from build123d import *

# Parameters (mm, degrees)
BOSS_EXTRUDE1_DEPTH                               = 3
CONVERT_SOLID1_DEPTH                              = 1
SKETCH8_R                                         = 2
CUT_EXTRUDE1_DEPTH                                = 2
CSK_FOR_4_FLAT_HEAD_MACHINE_SCREW_100_D           = 3.2639
CSK_FOR_4_FLAT_HEAD_MACHINE_SCREW_100_DEPTH       = 2
CSK_FOR_4_FLAT_HEAD_MACHINE_SCREW_100_CSINK_D     = 5.715
CSK_FOR_4_FLAT_HEAD_MACHINE_SCREW_100_CSINK_ANGLE = 100
CSK_FOR_4_FLAT_HEAD_MACHINE_SCREW_100_TIP         = 0.980574487


# Read off the part's stored shape, not the designer's step: Convert-Solid1
with BuildPart() as part:
    # Sketch2 → Boss-Extrude1 (new body)
    with BuildSketch(Plane(origin=(0, 0, 0), x_dir=(1, 0, 0), z_dir=(0, 1, 0))):
        with BuildLine():
            Line((-15.860247962, 17.20906431), (-13.637639272, 20.383278482))
            ThreePointArc((-13.637639272, 20.383278482), (-19.875283017, 22.35), (-26.112926762, 20.383278482))
            Line((-26.112926762, 20.383278482), (-26.112926762, 33.35))
            Line((-26.112926762, 33.35), (-26.112926762, 55.85))
            Line((-26.112926762, 55.85), (-16.112926762, 55.85))
            Line((-16.112926762, 55.85), (-16.112926762, 33.35))
            Line((-16.112926762, 33.35), (26.112926762, 33.35))
            Line((26.112926762, 33.35), (26.112926762, 20.383278482))
            ThreePointArc((26.112926762, 20.383278482), (19.875283017, 22.35), (13.637639272, 20.383278482))
            Line((13.637639272, 20.383278482), (15.860247962, 17.20906431))
            ThreePointArc((15.860247962, 17.20906431), (13.666207185, 14.707240293), (12.875283017, 11.475))
            ThreePointArc((12.875283017, 11.475), (10.092914311, 8.804356775), (6.237643745, 8.908278482))
            ThreePointArc((6.237643745, 8.908278482), (0, 10.875), (-6.237643745, 8.908278482))
            ThreePointArc((-6.237643745, 8.908278482), (-10.092914311, 8.804356775), (-12.875283017, 11.475))
            ThreePointArc((-12.875283017, 11.475), (-13.666207185, 14.707240293), (-15.860247962, 17.20906431))
        make_face()
    extrude(amount=BOSS_EXTRUDE1_DEPTH)

    # Convert-Solid1 outline → Convert-Solid1 (cut)
    with BuildSketch(Plane(origin=(0, 0, 0), x_dir=(1, 0, 0), z_dir=(0, 1, 0))):
        with BuildLine():
            Line((-26.112926762, 55.85), (-26.112926762, 20.383278482))
            ThreePointArc((-26.112926762, 20.383278482), (-19.875283017, 22.35), (-13.637639272, 20.383278482))
            Line((-13.637639272, 20.383278482), (-15.860247962, 17.20906431))
            ThreePointArc((-15.860247962, 17.20906431), (-13.666207185, 14.707240292), (-12.875283017, 11.475))
            ThreePointArc((-12.875283017, 11.475), (-10.092914311, 8.804356775), (-6.237643745, 8.908278482))
            ThreePointArc((-6.237643745, 8.908278482), (0, 10.875), (6.237643745, 8.908278482))
            ThreePointArc((6.237643745, 8.908278482), (10.092914311, 8.804356775), (12.875283017, 11.475))
            ThreePointArc((12.875283017, 11.475), (13.666207185, 14.707240292), (15.860247962, 17.20906431))
            Line((15.860247962, 17.20906431), (13.637639272, 20.383278482))
            ThreePointArc((13.637639272, 20.383278482), (19.875283017, 22.35), (26.112926762, 20.383278482))
            Line((26.112926762, 20.383278482), (26.112926762, 33.35))
            Line((26.112926762, 33.35), (-16.112926762, 33.35))
            Line((-16.112926762, 33.35), (-16.112926762, 55.85))
            Line((-16.112926762, 55.85), (-26.112926762, 55.85))
        make_face()
    extrude(amount=CONVERT_SOLID1_DEPTH, mode=Mode.SUBTRACT)

    # Sketch8 → Cut-Extrude1 (cut)
    with BuildSketch(Plane(origin=(0, 3, 0), x_dir=(1, 0, 0), z_dir=(0, 1, 0))):
        with Locations(Location((-21.112926762, 51.85, 0), (0, 0, 270))):
            Circle(SKETCH8_R)
        with Locations(Location((-21.112926762, 42.35, 0), (0, 0, 270))):
            Circle(SKETCH8_R)
    extrude(amount=-CUT_EXTRUDE1_DEPTH, mode=Mode.SUBTRACT)

    # CSK for #4 Flat Head Machine Screw (100)1
    with Locations(Plane(origin=(0, 3, 0), x_dir=(1, 0, 0), z_dir=(0, 1, 0))):
        with Locations((7.875283017, 28.35), (-7.875283017, 28.35)):
            CounterSinkHole(CSK_FOR_4_FLAT_HEAD_MACHINE_SCREW_100_D / 2, CSK_FOR_4_FLAT_HEAD_MACHINE_SCREW_100_CSINK_D / 2, depth=CSK_FOR_4_FLAT_HEAD_MACHINE_SCREW_100_DEPTH, counter_sink_angle=CSK_FOR_4_FLAT_HEAD_MACHINE_SCREW_100_CSINK_ANGLE)
            with Locations((0, 0, -(CSK_FOR_4_FLAT_HEAD_MACHINE_SCREW_100_DEPTH + CSK_FOR_4_FLAT_HEAD_MACHINE_SCREW_100_TIP / 2))):  # 118° drill point
                Cone(0, CSK_FOR_4_FLAT_HEAD_MACHINE_SCREW_100_D / 2, CSK_FOR_4_FLAT_HEAD_MACHINE_SCREW_100_TIP, mode=Mode.SUBTRACT)


solid = part.part
Part model, mm, in its own coordinate system. A direction names the side the tool comes from. Give positions to 0.01 mm unless a question says otherwise; leave off trailing zeros. Write each loop counter-clockwise with the first axis right and the second up, starting at its lowest first coordinate (ties: lowest second). Pieces come first, ordered by that corner, then holes.
1) Cut at D-D on z = -35.5. Write the cut outline in (x, y), then the cut area to 3 significant figures.
Resolved:
outline: (-26.11, 1) - (-16.11, 1) - (-16.11, 3) - (-26.11, 3) - close
area: 20.0 mm2
2) Probe L1, parallel to X at y = 1.65, z = -28.35; L2, parallel to X at y = 1.6, z = -42.35; L3, parallel to X at y = 1.45, z = -21.5. List the from-to ranges inside material, lowest first.
Resolved:
L1: x = -26.11 to -9.51, -6.24 to 6.24, 9.51 to 26.11
L2: x = -26.11 to -23.11, -19.11 to -16.11
L3: x = -26.11 to -24.09, -15.66 to 15.66, 24.09 to 26.11
3) Which spindle directions (+Z, -Z, +X, -X, +Y, -Y) get a long thin tool onto all of the face, cutting with end or side? Do faces 1 (the face through (5, 2, -33.35)), 2 (the face through (14.73, 1.99, -18.82)), 3 (the face through (10.145, 1.986, -8.825)), 4 (the face through (19.97, 1.99, -22.35)). Say none if no direction does.
Resolved:
face 1: -Z, +X, +Y, -Y
face 2: +X, +Y, -Y
face 3: +Z, +Y, -Y
face 4: +Y, -Y
4) Cut at C-C on x = 4. Write the cut outline in (y, z), then the cut area to 3 significant figures.
Resolved:
outline: (1, -33.35) - (3, -33.35) - (3, -10.11) - (1, -10.11) - close
area: 46.5 mm2
5) Cut at B-B on z = -28.35. Write the cut outline in (x, y), then the cut area to 3 significant figures.
Resolved:
outline: (-26.11, 1) - (-9.51, 1) - (-9.51, 1.97) - (-10.73, 3) - (-26.11, 3) - close; (-6.24, 1) - (6.24, 1) - (6.24, 1.97) - (5.02, 3) - (-5.02, 3) - (-6.24, 1.97) - close; (9.51, 1) - (26.11, 1) - (26.11, 3) - (10.73, 3) - (9.51, 1.97) - close
area: 88.9 mm2
6) Two-plate mould, pull along X, no slides. Class faces 5 (the face through (0, 3, -27)), 6 (the face through (-14.765, 1.986, -18.774)), 7 (the face through (8.229, 1.479, -26.757)): released by +X, released by -X, zero draft, split by the parting line, or undercut.
Resolved:
face 5: zero draft
face 6: released by -X
face 7: undercut
7) Pin check, flat tips, straight feed: pin 1 (1 mm diameter, centred on y = 1.5, z = -46.5, fed in from +X); pin 2 (1 mm diameter, centred on x = 18.5, y = 2.5, fed in from -Z); pin 3 (4 mm diameter, centred on x = -7.88, z = -28.35, fed in from +Y). Stop position of each tip, or through.
Resolved:
pin 1: stops at x = -16.11
pin 2: stops at z = -33.35
pin 3: stops at y = 2.28
8) Cut at A-A on z = -51.85. Write the cut outline in (x, y), then the cut area to 3 significant figures.
Resolved:
outline: (-26.11, 1) - (-23.11, 1) - (-23.11, 3) - (-26.11, 3) - close; (-19.11, 1) - (-16.11, 1) - (-16.11, 3) - (-19.11, 3) - close
area: 12.0 mm2
